```python
from build123d import *


with BuildPart() as part:
    # Sketch1 → Revolve1 (revolve)
    with BuildSketch(Plane(origin=(0, 0, 0), x_dir=(-1, 0, 0), z_dir=(0, 0, -1))):
        with BuildLine():
            Line((-2.3375, 11.1125), (-7.112, 11.1125))
            Line((-7.112, 11.1125), (-7.112, 9.906))
            Line((-7.112, 9.906), (-6.731, 9.906))
            Line((-6.731, 9.906), (-6.731, 6.625))
            Line((-6.731, 6.625), (-7.112, 6.625))
            Line((-7.112, 6.625), (-7.112, 5.125))
            Line((-7.112, 5.125), (0, 5.125))
            Line((0, 5.125), (0, 6.625))
            Line((0, 6.625), (-0.381, 6.625))
            Line((-0.381, 6.625), (-0.381, 9.906))
            Line((-0.381, 9.906), (0, 9.906))
            Line((0, 9.906), (0, 12.3063))
            Line((0, 12.3063), (-1.5875, 12.3063))
            Line((-1.5875, 12.3063), (-1.5875, 11.1125))
            ThreePointArc((-1.5875, 11.1125), (-1.7125, 10.895993649), (-1.9625, 10.895993649))
            Line((-1.9625, 10.895993649), (-2.3375, 11.1125))
        make_face()
    revolve(axis=Axis((7.112, 0, 0), (-1, 0, 0)))


solid = part.part
```
Read the model definition and answer for the solid it produces. Units are mm, in the model's axes. A direction names the side the tool comes from. Round coordinates to 2 decimals unless told otherwise and drop trailing zeros. Write each loop counter-clockwise with the first axis right and the second up, starting at its lowest first coordinate (ties: lowest second). Pieces come first, ordered by that corner, then holes. Notation, with made-up numbers: M 52.5,-36.5 L 97.5,-36.5 A24 ccw 97.5,-10.5 Z; hole C -5.5,27 d7. An arc over 180 degrees is marked long. One line per item, written item: value.
Q1. For a pull along Y with two mould halves and no side action, classify faces 4 (the cylindrical face through (0.8, -1.6, -12.2)), 5 (the flat face through (0.381, -6.5, 2.1)), 6 (the flat face through (7.112, -10, 2)) as +Y half, -Y half, draft (parallel to the pull), parting line (faces both ways), or undercut.
Data:
face 4: parting line
face 5: undercut
face 6: draft
Q2. Which of the six approach directions +Z, -Z, +X, -X, +Y, -Y give full straight-line access (tool end or side, diameter ignored) to faces 1 (the flat face through (7.112, 2, 5)), 2 (the cylindrical face through (0.193, 3.562, -5.586)), 3 (the cylindrical face through (6.92, -1.29, -9.82))?
Data:
face 1: +Z, -Z, +X, +Y, -Y
face 2: -X
face 3: +X
Q3. Straight lines are drawn through the part: line 1 (Z direction, x = 0.25, y = 0) (3 decimals); line 2 (Z direction, x = 7, y = 0) (1 decimal). For each, find the intervals that lie inside material, in ascending order. Write a range as [from, to].
Data:
line 1: [-12.306, -9.906], [-6.625, -5.125], [5.125, 6.625], [9.906, 12.306]
line 2: [-11.1, -9.9], [-6.6, -5.1], [5.1, 6.6], [9.9, 11.1]
Q4. Flat-ended cylindrical pins translate along their axes: pin 1 Ø8 at (y, z) = (0, 0) entering from +X; pin 2 Ø1 at (x, z) = (2, 1) entering from +Y; pin 3 Ø1.5 at (y, z) = (-7, 3.5) entering from -X. Find the tip coordinate at first contact, or state that the pin passes through.
Data:
pin 1: through
pin 2: y = 12.29
pin 3: x = 0.38
Q5. Find section D-D on x = 1. Write down the section's boundary in (y, z) (3 decimals).
Data:
outline: C 0,0 d24.613; hole C 0,0 d10.25
